```python
from build123d import *

# Parameters (mm, degrees)
SKETCH1_R           = 15.08125
BOSS_EXTRUDE1_DEPTH = 2.3114
BOSS_EXTRUDE1_DRAFT = -1
SKETCH7_R           = 15.08125
SKETCH7_R_2         = 13.30325
BOSS_EXTRUDE3_DEPTH = 6.35
BOSS_EXTRUDE3_DRAFT = -1
DRAFT1_ANGLE        = 10
FILLET2_R           = 0.381


with BuildPart() as part:
    # Sketch1 → Boss-Extrude1 (with draft: the straight prism first)
    with BuildSketch(Plane(origin=(0, 0, 0), x_dir=(1, 0, 0), z_dir=(0, 1, 0))):
        Circle(SKETCH1_R)
    extrude(amount=-BOSS_EXTRUDE1_DEPTH)
    # Boss-Extrude1: the draft: its side faces are tilted about the plane it starts from
    boss_extrude1_sides = [part.faces().sort_by_distance(p)[0] for p in [
        (-15.08125, -1.1557, 0),
    ]]
    draft(boss_extrude1_sides, Plane(origin=(0, 0, 0), x_dir=(1, 0, 0), z_dir=(0, 1, 0)), BOSS_EXTRUDE1_DRAFT)


with BuildPart() as boss_extrude3_tool:
    # Sketch7 → Boss-Extrude3 (with draft: the straight prism first)
    with BuildSketch(Plane(origin=(0, 0, 0), x_dir=(1, 0, 0), z_dir=(0, 1, 0))):
        Circle(SKETCH7_R)
        Circle(SKETCH7_R_2, mode=Mode.SUBTRACT)
    extrude(amount=-BOSS_EXTRUDE3_DEPTH)
    # Boss-Extrude3: the draft: its side faces are tilted about the plane it starts from
    boss_extrude3_sides = [boss_extrude3_tool.faces().sort_by_distance(p)[0] for p in [
        (-15.08125, -3.175, 0),
        (-13.30325, -3.175, 0),
    ]]
    draft(boss_extrude3_sides, Plane(origin=(0, 0, 0), x_dir=(1, 0, 0), z_dir=(0, 1, 0)), BOSS_EXTRUDE3_DRAFT)


with BuildPart() as part_1:
    add(part.part)

    # Boss-Extrude3: add boss_extrude3_tool
    add(boss_extrude3_tool.part)

    # Draft1
    draft1_faces = [part_1.faces().sort_by_distance(p)[0] for p in [
        (-13.37884265, -4.3307, 0),
    ]]
    draft(draft1_faces, Plane(origin=(0, -2.3114, 0), x_dir=(0, 0, -1), z_dir=(0, -1, 0)), DRAFT1_ANGLE)

    # Fillet2
    fillet2_edges = [part_1.edges().sort_by_distance(p)[0] for p in [
        (-14.970410338, -6.35, 0),
        (-14.055709781, -6.35, 0),
    ]]
    fillet(fillet2_edges, radius=FILLET2_R)


solid = part_1.part
```
For this review, take the finished solid that the model builds, in its own axes (mm). Round coordinates to 2 decimals unless told otherwise and drop trailing zeros. Loops run counter-clockwise (first coordinate to the right, second up) from the corner with the lowest first, then second, coordinate; pieces in that order, holes last.
(1) We need section A-A (y = -4). Give the boundary of the cut face in (x, z).
Returned:
outline: circle Ø30.02 at (0, 0); hole circle Ø27.28 at (0, 0)
(2) Clearance check with flat-ended pins moving along their axes: P1, Ø2, axis at x = -2, y = -2.5, coming from the +Z side; P2, Ø5, axis at x = 5.5, z = 5.5, coming from the -Y side; P3, Ø3, axis at x = 6.5, y = -5, coming from the +Z side; P4, Ø1, axis at x = -11.5, z = -11, coming from the +Y side. State where each tip first meets the part, or that it passes through.
Returned:
P1: stops at z = 15.01
P2: stops at y = -2.31
P3: stops at z = 14.14
P4: passes through
(3) Mouldability with a two-part tool opening along Z and no side actions: class faces 1 (the flat face through (0, 0, 0)), 2 (the conical face through (12.758, -2.492, -4.018)), 3 (the conical face through (-3.26, -2.95, 14.67)) as released by +Z, released by -Z, zero draft, split by the parting line, or undercut.
Returned:
face 1: zero draft
face 2: undercut
face 3: split by the parting line
(4) Wall thickness on line 1 along Z through (x, y) = (10, -4.5); line 2 along Z through (x, y) = (-10, -4.25); line 3 along Y through (x, z) = (-5.5, -6): over which ranges is each line inside the solid? List them lowest first.
Returned:
line 1: z = -11.18 to -9.41, 9.41 to 11.18
line 2: z = -11.19 to -9.34, 9.34 to 11.19
line 3: y = -2.31 to 0
